```python
from build123d import *

# Parameters (mm, degrees)
F0_R          = 3.25
F1_DEPTH      = 5
F2_R          = 2
F3_SIZE       = 2.25
F5_DEPTH      = 2
F5_DEPTH_BACK = 2


with BuildPart() as f1:
    # F0 (on Top) → F1 (new body)
    with BuildSketch(Plane.XY):
        with BuildLine():
            ThreePointArc((-37.6418413316, -26.8729284069), (-14.1089924944, 44.0454178184), (46.25, 0))
            ThreePointArc((46.25, 0), (21.1682493511, -41.121377888), (-26.8729284069, -37.6418413316))
            ThreePointArc((-26.8729284069, -37.6418413316), (-31.0817991261, -46.8950788332), (-41.0316193316, -48.9778834013))
            Line((-41.0316193316, -48.9778834013), (-10.3771158244, -57.212447804))
            ThreePointArc((-10.3771158244, -57.212447804), (0, -58.5819486205), (10.3771158244, -57.212447804))
            Line((10.3771158244, -57.212447804), (41.0316193316, -48.9778834013))
            ThreePointArc((41.0316193316, -48.9778834013), (46.6175743255, -45.4775418864), (49.2834994538, -39.44860109))
            Line((49.2834994538, -39.44860109), (53.4322534987, -4.7486065209))
            ThreePointArc((53.4322534987, -4.7486065209), (53.7151194618, 0), (53.4322534987, 4.7486065209))
            Line((53.4322534987, 4.7486065209), (49.2834994538, 39.44860109))
            ThreePointArc((49.2834994538, 39.44860109), (46.6175743255, 45.4775418864), (41.0316193316, 48.9778834013))
            Line((41.0316193316, 48.9778834013), (10.3771158244, 57.212447804))
            ThreePointArc((10.3771158244, 57.212447804), (0, 58.5819486205), (-10.3771158244, 57.212447804))
            Line((-10.3771158244, 57.212447804), (-41.0316193316, 48.9778834013))
            ThreePointArc((-41.0316193316, 48.9778834013), (-46.6175743255, 45.4775418864), (-49.2834994538, 39.44860109))
            Line((-49.2834994538, 39.44860109), (-53.4322534987, 4.7486065209))
            ThreePointArc((-53.4322534987, 4.7486065209), (-53.7151194618, 0), (-53.4322534987, -4.7486065209))
            Line((-53.4322534987, -4.7486065209), (-49.2834994538, -39.44860109))
            ThreePointArc((-49.2834994538, -39.44860109), (-46.3686757307, -30.4705928986), (-37.6418413316, -26.8729284069))
        make_face()
        with Locations((38.113055506, -38.113055506)):
            Circle(F0_R, mode=Mode.SUBTRACT)
        with Locations((-38.113055506, 38.113055506)):
            Circle(F0_R, mode=Mode.SUBTRACT)
        with Locations((38.113055506, 38.113055506)):
            Circle(F0_R, mode=Mode.SUBTRACT)
        with BuildLine():
            ThreePointArc((-26.8729284069, -37.6418413316), (-32.7036886299, -32.7036886299), (-37.6418413316, -26.8729284069))
            ThreePointArc((-37.6418413316, -26.8729284069), (-46.3686757307, -30.4705928986), (-49.2834994538, -39.44860109))
            ThreePointArc((-49.2834994538, -39.44860109), (-46.7245900781, -45.3521143062), (-41.3487870684, -48.8876803837))
            ThreePointArc((-41.3487870684, -48.8876803837), (-41.1905337069, -48.9339440057), (-41.0316193316, -48.9778834013))
            ThreePointArc((-41.0316193316, -48.9778834013), (-31.0817991261, -46.8950788332), (-26.8729284069, -37.6418413316))
        make_face()
        with Locations((-38.113055506, -38.113055506)):
            Circle(F0_R, mode=Mode.SUBTRACT)
    extrude(amount=F1_DEPTH)

    # F2
    f2_edges = [f1.edges().sort_by_distance(p)[0] for p in [
        (-25.704368, 53.095166, 5),
    ]]
    fillet(f2_edges, radius=F2_R)

    # F3
    f3_edges = [f1.edges().sort_by_distance(p)[0] for p in [
        (-41.363056, 38.113056, 5),
        (34.863056, 38.113056, 5),
        (34.863056, -38.113056, 5),
        (-41.363056, -38.113056, 5),
    ]]
    chamfer(f3_edges, length=F3_SIZE)

    # F4 (on Right) → F5 (cut, two sides)
    with BuildSketch(Plane.YZ) as f5_sk:
        Polygon((-58.5819486205, 0), (-57.212447804, 0), (-55.5819486205, 0), (-55.5819486205, 1), (-58.5819486205, 1), align=None)
    extrude(amount=-F5_DEPTH, mode=Mode.SUBTRACT)
    extrude(f5_sk.sketch, amount=F5_DEPTH_BACK, mode=Mode.SUBTRACT)


solid = f1.part
```
Source: CAD feature listing. Evaluate the final solid. Frame: model axes, mm. A direction names the side the tool comes from. Give positions to 0.01 mm unless a question says otherwise; leave off trailing zeros. Loops run counter-clockwise (first coordinate to the right, second up) from the corner with the lowest first, then second, coordinate; pieces in that order, holes last. Notation, with made-up numbers: (55, -2) - (95, -2) arc R16 cw to (95, 25) - close; hole circle Ø7 at (38, -23). An arc over 180 degrees is marked (long way). Use CSV: the item, a comma, the result in double quotes.
1) Cut plane A-A (x = 0). Output: boundary loops of the cut face in (y, z), and give its area (3 significant figures).
Worked out:
outline,"(-58.58, 1) - (-55.58, 1) - (-55.58, 0) - (-46.25, 0) - (-46.25, 5) - (-56.58, 5) arc R2 ccw to (-58.58, 3) - close; (46.25, 0) - (58.58, 0) - (58.58, 3) arc R2 ccw to (56.58, 5) - (46.25, 5) - close"
area,"119 mm^2"
2) Line query: line 1 (Y direction, x = 37, z = 3.7); line 2 (X direction, y = -39, z = 0.6); line 3 (Y direction, x = 39, z = 0.3). Output: solid intervals per line, ascending.
Worked out:
line 1,"y = -49.93 to -42.16, -34.06 to -27.75, 27.75 to 34.06, 42.16 to 49.93"
line 2,"x = -49.34 to -41.24, -34.99 to -24.86, 24.86 to 34.99, 41.24 to 49.34"
line 3,"y = -49.52 to -41.24, -34.99 to -24.86, 24.86 to 34.99, 41.24 to 49.52"
3) Mould query, pull axis X, two halves, no side actions, for faces 1 (the flat face through (-25.919, -53.038, 1.479)), 2 (the cylindrical face through (34.866, -37.97, 1.356)), 3 (the cylindrical face through (46.6, -45.5, 1.5)). Classes: +X half, -X half, draft (parallel to the pull), parting line (faces both ways), or undercut.
Worked out:
face 1,"-X half"
face 2,"undercut"
face 3,"+X half"
4) Pin query (flat end, axial travel): P1, Ø1, axis at x = -3.5, z = 1.5, coming from the -Y side; P2, Ø3, axis at y = 21.5, z = 2, coming from the -X side; P3, Ø1.5, axis at y = 0, z = 4, coming from the +X side. Return the tip coordinate at first contact, or that it passes through.
Worked out:
P1,"stops at y = -58.47"
P2,"stops at x = -51.61"
P3,"stops at x = 53.7"
5) Set-up query: faces 4 (the cylindrical face through (-41.36, 38.26, 1.36)), 5 (the flat face through (0, -57, 1)). Return all of +Z, -Z, +X, -X, +Y, -Y with unobstructed straight access to the full face (end or side cutting, diameter ignored); none if empty.
Worked out:
face 4,"+Z, -Z"
face 5,"-Z, -Y"
